from build123d import *

# Parameters (mm, degrees)
F0_W     = 203.2
F0_H     = 254
F1_DEPTH = 203.2
F2_T     = -12.7
F3_W     = 101.6
F3_H     = 203.2
F4_DEPTH = 25.4


with BuildPart() as f1:
    # F0 (on Top) → F1 (new body)
    with BuildSketch(Plane.XY):
        with Locations((-25.257506, 12.597671)):
            Rectangle(F0_W, F0_H)
    extrude(amount=F1_DEPTH)

    # F2
    f2_openings = [f1.faces().sort_by_distance(p)[0] for p in [
        (-25.257506, -114.402329, 101.6),
    ]]
    offset(amount=F2_T, openings=f2_openings)

    # F3 (on face) → F4 (join)
    with BuildSketch(Plane.XZ.offset(114.402329)):
        with Locations((-76.057506, 101.6)):
            Rectangle(F3_W, F3_H)
        with Locations((25.542494, 101.6)):
            Rectangle(F3_W, F3_H)
    extrude(amount=F4_DEPTH)


solid = f1.part
Verification items for the finished model (mm, model axes). A direction names the side the tool comes from. Coordinates: 2 decimals unless noted, no trailing zeros. Write each loop counter-clockwise with the first axis right and the second up, starting at its lowest first coordinate (ties: lowest second). Pieces come first, ordered by that corner, then holes. Notation, with made-up numbers: M 9,-27 L 61,-27 A7 ccw 61,-21 Z; hole C -18.5,17 d11. An arc over 180 degrees is marked long. Use a Markdown table: item, result.
Q1. Thickness scan on line 1 (Z direction, x = -49, y = 27); line 2 (X direction, y = -61, z = 147.5); line 3 (Y direction, x = -38.5, z = 67). Record the ranges inside material, lowest first.
Reply:
| item | result |
|---|---|
| line 1 | z = 0 to 12.7, 190.5 to 203.2 |
| line 2 | x = -126.86 to -114.16, 63.64 to 76.34 |
| line 3 | y = -139.8 to -114.4, 126.9 to 139.6 |
Q2. Sectioned sample at A-A, the plane x = -2. Record the boundary of the cut face in (y, z), plus the area to 3 significant figures.
Reply:
| item | result |
|---|---|
| outline | M -139.8,0 L 139.6,0 L 139.6,203.2 L -139.8,203.2 Z; hole M -114.4,12.7 L 126.9,12.7 L 126.9,190.5 L -114.4,190.5 Z |
| area | 13,900 mm² |
Q3. Sectioned sample at B-B, the plane z = 90.5. Record the boundary of the cut face in (x, y), plus the area to 3 significant figures.
Reply:
| item | result |
|---|---|
| outline | M -126.86,-139.8 L 76.34,-139.8 L 76.34,139.6 L -126.86,139.6 Z; hole M -114.16,-114.4 L 63.64,-114.4 L 63.64,126.9 L -114.16,126.9 Z |
| area | 13,900 mm² |
Q4. Draft check along X on faces 3 (the face through (-24, 2, 203.2)), 4 (the face through (-27, 8, 190.5)), 5 (the face through (-126.858, 2, 100)). Enter one of: +X half, -X half, draft (parallel to the pull), parting line (faces both ways), or undercut.
Reply:
| item | result |
|---|---|
| face 3 | draft |
| face 4 | undercut |
| face 5 | -X half |
Q5. Set-up check for faces 1 (the face through (-27, 139.598, 100)), 2 (the face through (-114.158, 5, 100)): record each of +Z, -Z, +X, -X, +Y, -Y from which the full face is reachable in a straight line by a thin tool's end or side.
Reply:
| item | result |
|---|---|
| face 1 | +Z, -Z, +X, -X, +Y |
| face 2 | none |
